Autodesk Fusion 360 part; units mm, degrees
sketch "Sketch1" plane through (0, 0, 0) normal (1, 0, 0) x (0, 0, -1)
  circle A0 centre (0, 0) radius 21
  dimension "d1" = 42
extrude "Extrude1" add sketch "Sketch1" along normal blind 3.2
sketch "Sketch2" plane through (3.2, 0, 0) normal (1, 0, 0) x (0, 0, -1)
  circle A0 centre (0, 0) radius 21
  circle A1 centre (0, 0) radius 19
  dimension "d4" = 38
extrude "Extrude2" add sketch "Sketch2" along normal blind 3.6 contours A1
sketch "Sketch3" plane through (6.8, 0, 0) normal (1, 0, 0) x (0, 0, -1)
  circle A0 centre (0, 0) radius 19
  circle A1 centre (0, 0) radius 21
  dimension "d7" = 42
extrude "Extrude3" add sketch "Sketch3" along normal blind 3.2 contours A0 | A1
fillet "Fillet1" radius 1.5 2 edges at (3.2, 6.8707, 17.7142) (6.8, -6.8707, 17.7142)
sketch "Sketch4" plane through (0, 0, 0) normal (-1, 0, 0) x (0, 0, 1)
  circle A0 centre (0, 0) radius 21
  circle A1 centre (0, 0) radius 28.9
  dimension "d11" = 57.8
extrude "Extrude4" add sketch "Sketch4" along normal blind 2.4 contours A0 | A1
sketch "Sketch5" plane through (0, 0, 0) normal (1, 0, 0) x (0, 0, -1)
  circle A0 centre (0, 0) radius 28.9
  circle A1 centre (0, 0) radius 21
  circle A2 centre (0, 0) radius 24.7
  dimension "d14" = 49.4
extrude "Extrude5" add sketch "Sketch5" along normal blind 1.8 contours A0
sketch "Sketch6" plane through (10, 0, 0) normal (1, 0, 0) x (0, 0, -1)
  circle A0 centre (0, 0) radius 21
  circle A1 centre (0, 0) radius 19
  circle A2 centre (0, 0) radius 16.6
  dimension "d17" = -2.4
extrude "Extrude6" cut sketch "Sketch6" against normal blind 10 contours A2
fillet "Fillet2" radius 1.2 1 edges at (10, -7.5939, 19.5789)
fillet "Fillet3" radius 1.6 1 edges at (-2.4, -10.4507, -26.9443)
fillet "Fillet4" radius 0.6 1 edges at (1.8, 8.9319, 23.0285)
equation "d4 = 41 mm - 3 mm"
Read the model definition and answer for the solid it produces. Units are mm, in the model's axes. A direction names the side the tool comes from. Give positions to 0.01 mm unless a question says otherwise; leave off trailing zeros. Write each loop counter-clockwise with the first axis right and the second up, starting at its lowest first coordinate (ties: lowest second). Pieces come first, ordered by that corner, then holes. Notation, with made-up numbers: (6.5, -21) -> (26.5, -21) arc R27 cw to (26.5, 5) -> close; hole circle Ø5 at (-6.5, 72.5). An arc over 180 degrees is marked (long way). Answer as a JSON object with one key per item and string values.
1) Section C-C on x = 6 is taken. Write down the section's boundary in (y, z).
Findings below:
{"outline": "circle Ø38.35 at (0, 0); hole circle Ø33.2 at (0, 0)"}
2) Straight lines are drawn through the part: probe 1 along Y at (x, z) = (0.7, 0); probe 2 along Y at (x, z) = (5, 0); probe 3 along Y at (x, z) = (1.25, 9.5). For each, find the intervals that lie inside material, in ascending order. Write a range as from..to.
Findings below:
{"probe 1": "y = -28.9..-24.7, -21..-16.6, 16.6..21, 24.7..28.9", "probe 2": "y = -19..-16.6, 16.6..19", "probe 3": "y = -27.29..-22.8, -18.73..-13.61, 13.61..18.73, 22.8..27.29"}
3) Flat-ended cylindrical pins translate along their axes: pin 1 Ø4 at (x, z) = (8.5, -10) entering from +Y; pin 2 Ø2 at (x, z) = (1.5, 18.5) entering from +Y; pin 3 Ø10 at (y, z) = (4.5, 6.5) entering from +X. Find the tip coordinate at first contact, or state that the pin passes through.
Findings below:
{"pin 1": "stops at y = 19.42", "pin 2": "stops at y = 23", "pin 3": "stops at x = 0"}
4) A tool of negligible diameter and unlimited length cuts with its end or side. For faces 4 (the flat face through (10, -10.2, 13.3)), 5 (the cylindrical face through (1.58, -6.31, -20.03)), 6 (the flat face through (6.8, -9.2, -18.6)), from which of +Z, -Z, +X, -X, +Y, -Y can it reach the whole face along a straight path? Write none if from no direction.
Findings below:
{"face 4": "+Z, -Z, +X, +Y, -Y", "face 5": "+X", "face 6": "none"}
5) For a pull along Z with two mould halves and no side action, classify faces 1 (the cylindrical face through (0.59, -7.42, -23.56)), 2 (the cylindrical face through (7.79, -6.31, -20.03)), 3 (the flat face through (-2.4, 0, 0)) as pulls with the +Z half, pulls with the -Z half, needs draft (parallel to the pull), parting line crosses it, or undercut.
Findings below:
{"face 1": "undercut", "face 2": "parting line crosses it", "face 3": "needs draft"}
